Can you work these out from the model? Positions are in its coordinate system, mm. A direction names the side the tool comes from. Coordinates: 2 decimals unless noted, no trailing zeros. Order: outer loops, then holes, each group sorted by start corner. A loop starts at its lowest first (then second) coordinate and runs counter-clockwise, first axis right, second up. Notation, with made-up numbers: (22, 45.5) -> (36, 45.5) arc R18 ccw to (36, 50.5) -> close; hole circle Ø4 at (15, 85.5). An arc over 180 degrees is marked (long way). Answer as CSV lines item,"result".
from build123d import *

# Parameters (mm, degrees)
SKETCH1_R           = 1
BOSS_EXTRUDE1_DEPTH = 4.5
SKETCH2_R           = 1.75
BOSS_EXTRUDE2_DEPTH = 1
CHAMFER1_SIZE       = 0.2
SKETCH3_R           = 1.75
BOSS_EXTRUDE3_DEPTH = 1
CHAMFER2_SIZE       = 0.2


with BuildPart() as part:
    # Sketch1 → Boss-Extrude1 (new body)
    with BuildSketch(Plane(origin=(0, 0, 0), x_dir=(1, 0, 0), z_dir=(0, 1, 0))):
        Circle(SKETCH1_R)
    extrude(amount=BOSS_EXTRUDE1_DEPTH)

    # Sketch2 → Boss-Extrude2 (add)
    with BuildSketch(Plane(origin=(0, 4.5, 0), x_dir=(1, 0, 0), z_dir=(0, 1, 0))):
        Circle(SKETCH2_R)
    extrude(amount=BOSS_EXTRUDE2_DEPTH)

    # Chamfer1
    chamfer1_edges = [part.edges().sort_by_distance(p)[0] for p in [
        (-1.75, 5.5, 0),
    ]]
    chamfer(chamfer1_edges, length=CHAMFER1_SIZE)

    # Sketch3 → Boss-Extrude3 (add)
    with BuildSketch(Plane.XZ):
        Circle(SKETCH3_R)
    extrude(amount=BOSS_EXTRUDE3_DEPTH)

    # Chamfer2
    chamfer2_edges = [part.edges().sort_by_distance(p)[0] for p in [
        (-1.75, -1, 0),
    ]]
    chamfer(chamfer2_edges, length=CHAMFER2_SIZE)


solid = part.part
Q1. Imagine slicing it at D-D (y = 5). List the corners of the cut face in (x, z) for me.
Solution:
outline,"circle Ø3.5 at (0, 0)"
Q2. Imagine slicing it at B-B (x = 0). List the corners of the cut face in (y, z) for me, and give its area (3 significant figures).
Solution:
outline,"(-1, -1.55) -> (-0.8, -1.75) -> (0, -1.75) -> (0, -1) -> (4.5, -1) -> (4.5, -1.75) -> (5.3, -1.75) -> (5.5, -1.55) -> (5.5, 1.55) -> (5.3, 1.75) -> (4.5, 1.75) -> (4.5, 1) -> (0, 1) -> (0, 1.75) -> (-0.8, 1.75) -> (-1, 1.55) -> close"
area,"15.9 mm2"
Q3. Which directions (+Z, -Z, +X, -X, +Y, -Y) give clear straight access to the entire face, cutting with the end or side of a thin tool? Please do faces 1 (the flat face through (1, 0, -1)), 2 (the cylindrical face through (1.617, 4.894, 0.67)).
Solution:
face 1,"none"
face 2,"+Y, -Y"
Q4. Imagine slicing it at A-A (z = 0). List the corners of the cut face in (x, y) for me.
Solution:
outline,"(-1.75, -0.8) -> (-1.55, -1) -> (1.55, -1) -> (1.75, -0.8) -> (1.75, 0) -> (1, 0) -> (1, 4.5) -> (1.75, 4.5) -> (1.75, 5.3) -> (1.55, 5.5) -> (-1.55, 5.5) -> (-1.75, 5.3) -> (-1.75, 4.5) -> (-1, 4.5) -> (-1, 0) -> (-1.75, 0) -> close"
Q5. Imagine slicing it at C-C (y = 3). List the corners of the cut face in (x, z) for me.
Solution:
outline,"circle Ø2 at (0, 0)"
Q6. We'd pull the mould along Y, two halves only. Please class faces 3 (the flat face through (0, -1, 0)), 4 (the cylindrical face through (1.617, -0.394, -0.67)), 5 (the cylindrical face through (0, 2, 1)): pulls with the +Y half, pulls with the -Y half, needs draft (parallel to the pull), parting line crosses it, or undercut.
Solution:
face 3,"pulls with the -Y half"
face 4,"needs draft"
face 5,"undercut"
Q7. If I drill on line 1 (Y direction, x = 1.2, z = 0.1); line 2 (Y direction, x = 1.3, z = -1.05); line 3 (X direction, y = -0.5, z = 0.95), over which ranges is the centre line in solid material (lowest first)?
Solution:
line 1,"-1 to 0, 4.5 to 5.5"
line 2,"-0.88 to 0, 4.5 to 5.38"
line 3,"-1.47 to 1.47"
